from build123d import *

# Parameters (mm, degrees)
SKETCH1_R           = 9.525
BOSS_EXTRUDE1_DEPTH = 36
SKETCH2_R           = 25.4
BOSS_EXTRUDE2_DEPTH = 3.175
SKETCH3_R           = 4.7625
BOSS_EXTRUDE3_DEPTH = 12.7
SKETCH4_R           = 2.15265
CUT_EXTRUDE1_DEPTH  = 19.05
FILLET1_R           = 3
SKETCH5_W           = 3
SKETCH5_H           = 1.491900756
BOSS_EXTRUDE4_DEPTH = 10.6


with BuildPart() as part:
    # Sketch1 → Boss-Extrude1 (new body)
    with BuildSketch(Plane.XY):
        Circle(SKETCH1_R)
        with BuildLine():
            Line((-1.5, 5.2), (1.5, 5.2))
            Line((1.5, 5.2), (1.5, 3.708099244))
            ThreePointArc((1.5, 3.708099244), (0, -4), (-1.5, 3.708099244))
            Line((-1.5, 3.708099244), (-1.5, 5.2))
        make_face(mode=Mode.SUBTRACT)
    extrude(amount=BOSS_EXTRUDE1_DEPTH)

    # Sketch2 → Boss-Extrude2 (add)
    with BuildSketch(Plane.XY.offset(36)):
        Circle(SKETCH2_R)
    extrude(amount=BOSS_EXTRUDE2_DEPTH)

    # Sketch3 → Boss-Extrude3 (add)
    with BuildSketch(Plane.XY.offset(39.175)):
        Circle(SKETCH3_R)
    extrude(amount=BOSS_EXTRUDE3_DEPTH)

    # Sketch4 → Cut-Extrude1 (cut)
    with BuildSketch(Plane.XY.offset(39.175)):
        with Locations((0, 19.05)):
            Circle(SKETCH4_R)
        with Locations((13.470384182, 13.470384182)):
            Circle(SKETCH4_R)
        with Locations((19.05, 0)):
            Circle(SKETCH4_R)
        with Locations((13.470384182, -13.470384182)):
            Circle(SKETCH4_R)
        with Locations((-19.05, 0)):
            Circle(SKETCH4_R)
        with Locations((0, -19.05)):
            Circle(SKETCH4_R)
        with Locations((-13.470384182, -13.470384182)):
            Circle(SKETCH4_R)
        with Locations((-13.470384182, 13.470384182)):
            Circle(SKETCH4_R)
    extrude(amount=-CUT_EXTRUDE1_DEPTH, mode=Mode.SUBTRACT)

    # Fillet1
    fillet1_edges = [part.edges().sort_by_distance(p)[0] for p in [
        (-4.7625, 0, 39.175),
    ]]
    fillet(fillet1_edges, radius=FILLET1_R)

    # Sketch5 → Boss-Extrude4 (add)
    with BuildSketch(Plane(origin=(0, 0, 36), x_dir=(-1, 0, 0), z_dir=(0, 0, -1))):
        with Locations((0, 4.454049622)):
            Rectangle(SKETCH5_W, SKETCH5_H)
    extrude(amount=BOSS_EXTRUDE4_DEPTH)


solid = part.part
Can you work these out from the model? Positions are in its coordinate system, mm. A direction names the side the tool comes from. Give positions to 0.01 mm unless a question says otherwise; leave off trailing zeros. Loops run counter-clockwise (first coordinate to the right, second up) from the corner with the lowest first, then second, coordinate; pieces in that order, holes last. Notation, with made-up numbers: M 58,-18.75 L 80,-18.75 A15 cw 80,0.25 Z; hole C 69,-17 d2. An arc over 180 degrees is marked long. One line per item, written item: value. Start each with the question number.
1) If we section it at A-A, the plane x = 0: Write out the boundary of the cut face in (y, z) (1 decimal), and give its area (3 significant figures).
2) I'm going to push flat-ended pins straight in: pin 1 (7 mm diameter, centred on x = 19.05, y = 0, fed in from -Z); pin 2 (1.2 mm diameter, centred on y = 5, z = 17.5, fed in from +X); pin 3 (8 mm diameter, centred on y = -15.5, z = 23.5, fed in from +X); pin 4 (8 mm diameter, centred on x = 9.5, y = 7, fed in from +Z) (3 decimals). Where does each tip first touch, or does it pass through?
3) If we section it at C-C, the plane z = 23: Write out the boundary of the cut face in (x, y) (3 decimals).
4) Thinking about a two-plate mould opening in Y: for faces 1 (the face through (0, 0, 36)), 2 (the face through (-5.506, -24.796, 37.565)), 3 (the face through (2, -4, 0)), which applies, +Y half, -Y half, draft (parallel to the pull), parting line (faces both ways), or undercut?
5) If we section it at B-B, the plane y = 0: Write out the boundary of the cut face in (x, z) (1 decimal).
6) If we section it at D-D, the plane y = 19.05: Write out the boundary of the cut face in (x, z) (3 decimals).
7) On a 3-axis mill with a long thin cutter (end or side, diameter ignored), from which of +Z, -Z, +X, -X, +Y, -Y can I reach the whole of each face in a straight line? I mean faces 4 (the face through (0, 4, 25.4)), 5 (the face through (14.46, -15.38, 37.61)), 6 (the face through (5.3, 6, 39.175)). Say none if no direction works.
8) If I drill on line 1 (Y direction, x = 0, z = 37); line 2 (Z direction, x = -14, y = 3) (3 decimals); line 3 (X direction, y = 15, z = 36.5), over which ranges is the centre line in solid material (lowest first)? Write a range as [from, to].
Completed:
1. outline: M -25.4,36 L -21.2,36 L -21.2,39.2 L -25.4,39.2 Z; M -16.9,36 L -9.5,36 L -9.5,0 L -4,0 L -4,36 L 3.7,36 L 3.7,25.4 L 5.2,25.4 L 5.2,0 L 9.5,0 L 9.5,36 L 16.9,36 L 16.9,39.2 L 7.8,39.2 A3 cw 4.8,42.2 L 4.8,51.9 L -4.8,51.9 L -4.8,42.2 A3 cw -7.8,39.2 L -16.9,39.2 Z; M 21.2,36 L 25.4,36 L 25.4,39.2 L 21.2,39.2 Z
1. area: 629 mm^2
2. pin 1: stops at z = 36
2. pin 2: stops at x = 8.45
2. pin 3: passes through
2. pin 4: stops at z = 39.175
3. outline: C 0,0 d19.05; hole M -1.5,3.708 A4 ccw long 1.5,3.708 L 1.5,5.2 L -1.5,5.2 Z
4. face 1: undercut
4. face 2: parting line
4. face 3: draft
5. outline: M -25.4,36 L -21.2,36 L -21.2,39.2 L -25.4,39.2 Z; M -16.9,36 L -9.5,36 L -9.5,0 L -4,0 L -4,36 L 4,36 L 4,0 L 9.5,0 L 9.5,36 L 16.9,36 L 16.9,39.2 L 7.8,39.2 A3 cw 4.8,42.2 L 4.8,51.9 L -4.8,51.9 L -4.8,42.2 A3 cw -7.8,39.2 L -16.9,39.2 Z; M 21.2,36 L 25.4,36 L 25.4,39.2 L 21.2,39.2 Z
6. outline: M -16.801,36 L -2.153,36 L -2.153,39.175 L -16.801,39.175 Z; M 2.153,36 L 16.801,36 L 16.801,39.175 L 2.153,39.175 Z
7. face 4: -Z
7. face 5: +Z, -Z
7. face 6: +Z
8. line 1: y = [-25.4, -21.2], [-16.9, 16.9], [21.2, 25.4]
8. line 2: z = [36, 39.175]
8. line 3: x = [-20.5, -14.99], [-11.96, 11.96], [14.99, 20.5]
